Input: part model. Units: mm. Frame: model coordinates. A direction names the side the tool comes from. Coordinates: 2 decimals unless noted, no trailing zeros. Loops run counter-clockwise (first coordinate to the right, second up) from the corner with the lowest first, then second, coordinate; pieces in that order, holes last.
Item 1: Reachability of faces 1 (the flat face through (3, -2.5, 4)), 2 (the flat face through (-3, 2.5, 4)), 3 (the flat face through (0, 0, 0)), 4 (the flat face through (9.23, -0.04, 5.6)), 5 (the flat face through (4.55, 0, 6)) from +Z, -Z, +X, -X, +Y, -Y: full face, straight path, thin tool, end or side. Return the list, or none.
Item 2: Ray query, line 1 along X through (y, z) = (-0.25, 4); line 2 along Y through (x, z) = (-9.75, 3.5); line 3 along Z through (x, y) = (-0.15, -0.2). Return the intervals inside material, ascending.
Item 3: Pull-direction query (X, two-part tool) for faces 6 (the flat face through (-3.77, -0.04, 5.6)), 7 (the flat face through (-3.04, -0.04, 5.57)), 8 (the cylindrical face through (11.115, -5.599, 0.507)), 9 (the flat face through (-9, 2.5, 4)); classes: released by +X, released by -X, zero draft, split by the parting line, or undercut.
Item 4: Section B-B on z = 5.5. Return loops of the section in (x, y).
Item 5: Contact query for flat-ended pins moving along their axis: P1, Ø2, axis at x = -8, z = 3.5, coming from the -Y side; P2, Ø1.2, axis at y = 1, z = 6, coming from the -X side; P3, Ø1.6, axis at y = -1, z = 5.5, coming from the +X side. Output: stop coordinate, or through.
Item 6: Section A-A on z = 2.5. Return loops of the section in (x, y), and give its area (3 significant figures).
Item 7: Section D-D on x = 7.75. Return loops of the section in (y, z), and give its area (3 significant figures).
```python
from build123d import *

# Parameters (mm, degrees)
SKETCH1_W           = 22.8
SKETCH1_H           = 11.8
BOSS_EXTRUDE1_DEPTH = 1
BOSS_EXTRUDE2_DEPTH = 2.5
LPATTERN2_COUNT     = 3
LPATTERN2_PITCH     = 6.5
FILLET1_R           = 1
FILLET2_R           = 1


with BuildPart() as part:
    # Sketch1 → Boss-Extrude1 (new body)
    with BuildSketch(Plane.XY):
        Rectangle(SKETCH1_W, SKETCH1_H)
    extrude(amount=BOSS_EXTRUDE1_DEPTH)

    # Sketch3 → Boss-Extrude2 (add, symmetric)
    with BuildSketch(Plane.XZ):
        with BuildLine():
            Line((-9.9, 1), (-9.9, 4.581665383))
            Line((-9.9, 4.581665383), (-9.172059531, 6.581665383))
            Line((-9.172059531, 6.581665383), (-8.45, 6.581665383))
            Line((-8.45, 6.581665383), (-8.45, 5.081665383))
            ThreePointArc((-8.45, 5.081665383), (-6.65, 1.9), (-4.85, 5.081665383))
            Line((-4.85, 5.081665383), (-4.85, 6.581665383))
            Line((-4.85, 6.581665383), (-4.127940469, 6.581665383))
            Line((-4.127940469, 6.581665383), (-3.4, 4.581665383))
            Line((-3.4, 4.581665383), (-3.4, 1))
            Line((-3.4, 1), (-9.9, 1))
        make_face()
    boss_extrude2 = extrude(amount=BOSS_EXTRUDE2_DEPTH, both=True)

    # LPattern2: Boss-Extrude2 ×3
    with Locations(*[(i * LPATTERN2_PITCH, 0, 0) for i in range(1, LPATTERN2_COUNT)]):
        add(boss_extrude2)

    # Fillet1
    fillet1_edges = [part.edges().sort_by_distance(p)[0] for p in [
        (-11.4, 5.9, 0.5),
        (11.4, 5.9, 0.5),
        (11.4, -5.9, 0.5),
        (-11.4, -5.9, 0.5),
    ]]
    fillet(fillet1_edges, radius=FILLET1_R)

    # Fillet2
    fillet2_edges = [part.edges().sort_by_distance(p)[0] for p in [
        (-0.15, 2.5, 1),
        (-9.9, 0, 1),
        (-0.15, -2.5, 1),
        (9.6, 0, 1),
    ]]
    fillet(fillet2_edges, radius=FILLET2_R)


solid = part.part
```
Results found:
1. face 1: +Z, +X, -X, -Y
1. face 2: +Z, +X, -X, +Y
1. face 3: -Z, +X, -X, +Y, -Y
1. face 4: +Z, +X, +Y, -Y
1. face 5: +Z, +Y, -Y
2. line 1: x = -9.9 to -8.75, -4.55 to -2.25, 1.95 to 4.25, 8.45 to 9.6
2. line 2: y = -2.5 to 2.5
2. line 3: z = 0 to 1.9
3. face 6: undercut
3. face 7: undercut
3. face 8: released by +X
3. face 9: zero draft
4. outline: (-9.57, -2.5) - (-8.45, -2.5) - (-8.45, 2.5) - (-9.57, 2.5) - close; (-4.85, -2.5) - (-3.73, -2.5) - (-3.73, 2.5) - (-4.85, 2.5) - close; (-3.07, -2.5) - (-1.95, -2.5) - (-1.95, 2.5) - (-3.07, 2.5) - close; (1.65, -2.5) - (2.77, -2.5) - (2.77, 2.5) - (1.65, 2.5) - close; (3.43, -2.5) - (4.55, -2.5) - (4.55, 2.5) - (3.43, 2.5) - close; (8.15, -2.5) - (9.27, -2.5) - (9.27, 2.5) - (8.15, 2.5) - close
5. P1: stops at y = -2.5
5. P2: stops at x = -9.6
5. P3: stops at x = 9.56
6. outline: (-9.9, -2.5) - (-8.12, -2.5) - (-8.12, 2.5) - (-9.9, 2.5) - close; (-5.18, -2.5) - (-1.62, -2.5) - (-1.62, 2.5) - (-5.18, 2.5) - close; (1.32, -2.5) - (4.88, -2.5) - (4.88, 2.5) - (1.32, 2.5) - close; (7.82, -2.5) - (9.6, -2.5) - (9.6, 2.5) - (7.82, 2.5) - close
6. area: 53.4 mm2
7. outline: (-5.9, 0) - (5.9, 0) - (5.9, 1) - (3.5, 1) arc R1 cw to (2.5, 2) - (2.5, 2.43) - (-2.5, 2.43) - (-2.5, 2) arc R1 cw to (-3.5, 1) - (-5.9, 1) - close
7. area: 19.4 mm2
